Input: dimensioned drawing with shaded views. Units: mm. Origin: part minimum x, y, z. Round coordinates to 2 decimals unless told otherwise and drop trailing zeros. Write each loop counter-clockwise with the first axis right and the second up, starting at its lowest first coordinate (ties: lowest second). Pieces come first, ordered by that corner, then holes. Notation, with made-up numbers: (-6, 82.5) - (16, 82.5) arc R16 ccw to (16, 108.5) - close; hole circle Ø9 at (-38.5, 48). An arc over 180 degrees is marked (long way). Use one line per item in the form item = value.
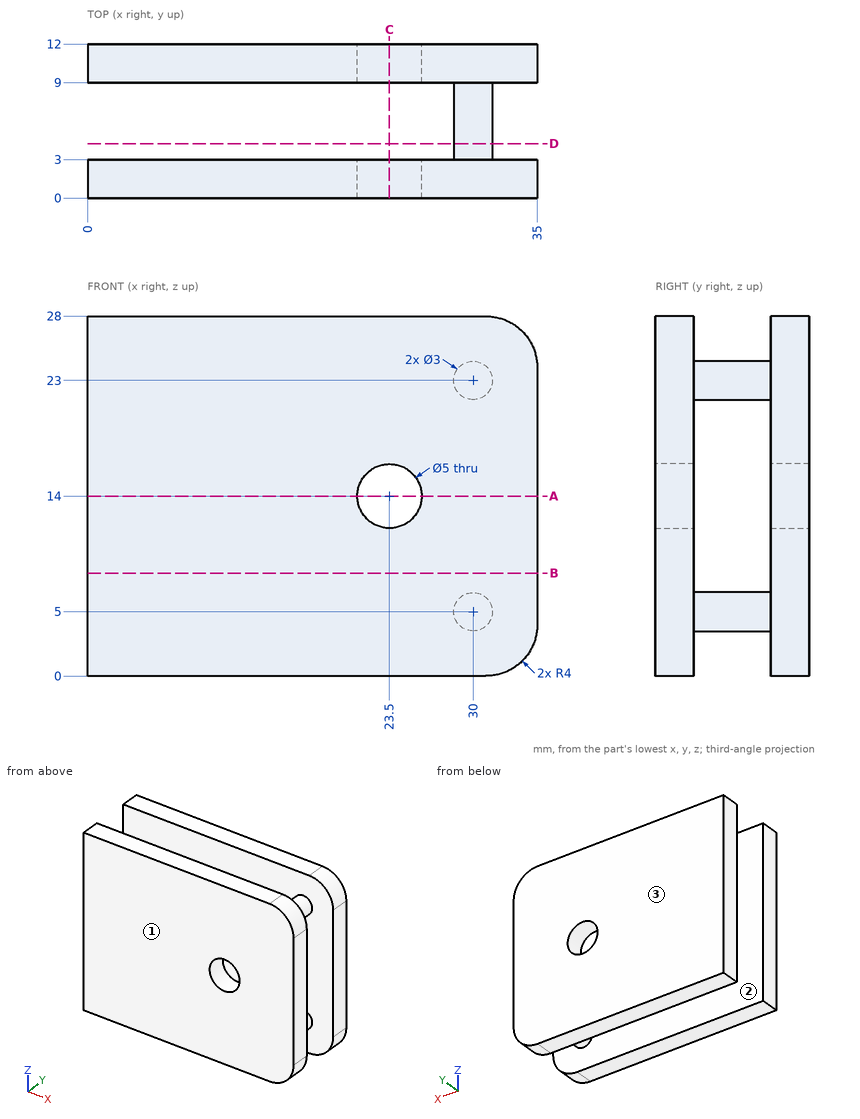
(1) Cut plane B-B on z = 8. Output: boundary loops of the cut face in (x, y), then the cut area to 3 significant figures.
Derived:
outline = (0, 0) - (35, 0) - (35, 3) - (0, 3) - close; (0, 9) - (35, 9) - (35, 12) - (0, 12) - close
area = 210 mm^2
(2) Material intervals for L1, parallel to Y at x = 2, z = 3.25; L2, parallel to X at y = 10.9, z = 14; L3, parallel to Z at x = 23.5, y = 11.15, sorted ascending.
Derived:
L1 = 0 to 3, 9 to 12
L2 = 0 to 21, 26 to 35
L3 = 0 to 11.5, 16.5 to 28
(3) First-contact query: pin 1 Ø3 at (x, z) = (23.5, 14) entering from -Y; pin 2 Ø1.5 at (y, z) = (7, 4.5) entering from -X. Flat tips, straight axial feed; report the tip coordinate or a pass-through.
Derived:
pin_1 = through
pin_2 = 28.5
(4) Cut plane A-A on z = 14. Output: boundary loops of the cut face in (x, y).
Derived:
outline = (0, 0) - (21, 0) - (21, 3) - (0, 3) - close; (0, 9) - (21, 9) - (21, 12) - (0, 12) - close; (26, 0) - (35, 0) - (35, 3) - (26, 3) - close; (26, 9) - (35, 9) - (35, 12) - (26, 12) - close
(5) Cut plane C-C on x = 23.5. Output: boundary loops of the cut face in (y, z), then the cut area to 3 significant figures.
Derived:
outline = (0, 0) - (3, 0) - (3, 11.5) - (0, 11.5) - close; (0, 16.5) - (3, 16.5) - (3, 28) - (0, 28) - close; (9, 0) - (12, 0) - (12, 11.5) - (9, 11.5) - close; (9, 16.5) - (12, 16.5) - (12, 28) - (9, 28) - close
area = 138 mm^2
(6) Cut plane D-D on y = 4.25. Output: boundary loops of the cut face in (x, z), then the cut area to 3 significant figures.
Derived:
outline = circle Ø3 at (30, 5); circle Ø3 at (30, 23)
area = 14.1 mm^2
(7) Draft query along Y for the marked faces 1, 2 and 3. Return one class per face: released by +Y, released by -Y, zero draft, split by the parting line, or undercut.
Derived:
face_1 = released by -Y
face_2 = undercut
face_3 = released by +Y
